Geometry: final body of the model. Coordinates: model frame, mm. A direction names the side the tool comes from. Coordinates: 2 decimals unless noted, no trailing zeros. Use CSV: the item, a comma, the result in double quotes. Start each with the question number.
Q1. Section query A-A, the plane y = -31. State how many separate pieces and enclosed holes the cut face has, and give its area (3 significant figures).
Q2. Mould query, pull axis X, two halves, no side actions, for faces 1 (the face through (3, 0, -3)), 2 (the face through (-67.5, -50, 2)), 3 (the face through (0, -10, 180)). Classes: +X half, -X half, draft (parallel to the pull), parting line (faces both ways), or undercut.
Q3. First-contact query: P1, Ø10, axis at y = -49.5, z = -59, coming from the -X side; P2, Ø18, axis at y = -44.5, z = -43, coming from the -X side; P3, Ø1.5, axis at x = 0.5, y = -54.5, coming from the -Z side. Flat tips, straight axial feed; report the tip coordinate or a pass-through.
Q4. Ray query, probe 1 along X at (y, z) = (-11.75, 0); probe 2 along X at (y, z) = (-9, -170). Return the intervals inside material, ascending.
Q5. Access query for faces 4 (the face through (-10, -10, -166)), 5 (the face through (-130.156, -49.58, 58.015)), 6 (the face through (87.5, -50, 2)), 7 (the face through (105.106, -9.86, -107.018)). Directions: +Z, -Z, +X, -X, +Y, -Y. A direction counts if a zero-diameter tool reaches every point of the face in a straight line with its end or side. Return the directions, or none.
from build123d import *

# Parameters (mm, degrees)
SKETCH3_R           = 5
BOSS_EXTRUDE4_DEPTH = 20
SKETCH4_W           = 5
SKETCH4_H           = 260
BOSS_EXTRUDE5_DEPTH = 60


with BuildPart() as part:
    # Sketch3 → Boss-Extrude4 (new body)
    with BuildSketch(Plane(origin=(0, 0, 0), x_dir=(1, 0, 0), z_dir=(0, 1, 0))):
        with BuildLine():
            Line((161.369142032, 10), (170, 10))
            ThreePointArc((170, 10), (180, 0), (170, -10))
            Line((170, -10), (161.369142032, -10))
            ThreePointArc((161.369142032, -10), (152.849946816, -13.180462695), (148.499210458, -21.165644172))
            ThreePointArc((148.499210458, -21.165644172), (106.066017178, -106.066017178), (21.165644172, -148.499210458))
            ThreePointArc((21.165644172, -148.499210458), (13.180462695, -152.849946816), (10, -161.369142032))
            Line((10, -161.369142032), (10, -170))
            ThreePointArc((10, -170), (0, -180), (-10, -170))
            Line((-10, -170), (-10, -161.369142032))
            ThreePointArc((-10, -161.369142032), (-13.180462695, -152.849946816), (-21.165644172, -148.499210458))
            ThreePointArc((-21.165644172, -148.499210458), (-106.066017178, -106.066017178), (-148.499210458, -21.165644172))
            ThreePointArc((-148.499210458, -21.165644172), (-152.849946816, -13.180462695), (-161.369142032, -10))
            Line((-161.369142032, -10), (-170, -10))
            ThreePointArc((-170, -10), (-180, 0), (-170, 10))
            Line((-170, 10), (-161.369142032, 10))
            ThreePointArc((-161.369142032, 10), (-152.849946816, 13.180462695), (-148.499210458, 21.165644172))
            ThreePointArc((-148.499210458, 21.165644172), (-106.066017178, 106.066017178), (-21.165644172, 148.499210458))
            ThreePointArc((-21.165644172, 148.499210458), (-13.180462695, 152.849946816), (-10, 161.369142032))
            Line((-10, 161.369142032), (-10, 170))
            ThreePointArc((-10, 170), (0, 180), (10, 170))
            Line((10, 170), (10, 161.369142032))
            ThreePointArc((10, 161.369142032), (13.180462695, 152.849946816), (21.165644172, 148.499210458))
            ThreePointArc((21.165644172, 148.499210458), (106.066017178, 106.066017178), (148.499210458, 21.165644172))
            ThreePointArc((148.499210458, 21.165644172), (152.849946816, 13.180462695), (161.369142032, 10))
        make_face()
        with Locations((0, 170)):
            Circle(SKETCH3_R, mode=Mode.SUBTRACT)
        with Locations((170, 0)):
            Circle(SKETCH3_R, mode=Mode.SUBTRACT)
        with Locations((0, -170)):
            Circle(SKETCH3_R, mode=Mode.SUBTRACT)
        with Locations((-170, 0)):
            Circle(SKETCH3_R, mode=Mode.SUBTRACT)
    extrude(amount=-BOSS_EXTRUDE4_DEPTH)

    # Sketch4 → Boss-Extrude5 (add)
    with BuildSketch(Plane(origin=(0, -20, 0), x_dir=(1, 0, 0), z_dir=(0, 1, 0))):
        Rectangle(SKETCH4_W, SKETCH4_H)
        with Locations((10, 0)):
            Rectangle(SKETCH4_W, SKETCH4_H)
        with Locations((20, 0)):
            Rectangle(SKETCH4_W, SKETCH4_H)
        with Locations((30, 0)):
            Rectangle(SKETCH4_W, SKETCH4_H)
        with Locations((40, 0)):
            Rectangle(SKETCH4_W, SKETCH4_H)
        with Locations((50, 0)):
            Rectangle(SKETCH4_W, SKETCH4_H)
        with Locations((60, 0)):
            Rectangle(SKETCH4_W, SKETCH4_H)
        with Locations((70, 0)):
            Rectangle(SKETCH4_W, SKETCH4_H)
        with BuildLine():
            Line((82.5, 116.189500386), (82.5, -116.189500386))
            ThreePointArc((82.5, -116.189500386), (80.017987314, -117.912559578), (77.5, -119.582607431))
            Line((77.5, -119.582607431), (77.5, 119.582607431))
            ThreePointArc((77.5, 119.582607431), (80.017987314, 117.912559578), (82.5, 116.189500386))
        make_face()
        with BuildLine():
            Line((92.5, 108.397416943), (92.5, -108.397416943))
            ThreePointArc((92.5, -108.397416943), (90.023058171, -110.463111478), (87.5, -112.472218792))
            Line((87.5, -112.472218792), (87.5, 112.472218792))
            ThreePointArc((87.5, 112.472218792), (90.023058171, 110.463111478), (92.5, 108.397416943))
        make_face()
        with BuildLine():
            Line((102.5, 98.994949366), (102.5, -98.994949366))
            ThreePointArc((102.5, -98.994949366), (100.030353094, -101.489794856), (97.5, -103.923048454))
            Line((97.5, -103.923048454), (97.5, 103.923048454))
            ThreePointArc((97.5, 103.923048454), (100.030353094, 101.489794856), (102.5, 98.994949366))
        make_face()
        with BuildLine():
            Line((112.5, 87.464278423), (112.5, -87.464278423))
            ThreePointArc((112.5, -87.464278423), (110.041959984, -90.537379258), (107.5, -93.541434669))
            Line((107.5, -93.541434669), (107.5, 93.541434669))
            ThreePointArc((107.5, 93.541434669), (110.041959984, 90.537379258), (112.5, 87.464278423))
        make_face()
        with Locations((-10, 0)):
            Rectangle(SKETCH4_W, SKETCH4_H)
        with Locations((-20, 0)):
            Rectangle(SKETCH4_W, SKETCH4_H)
        with Locations((-30, 0)):
            Rectangle(SKETCH4_W, SKETCH4_H)
        with Locations((-40, 0)):
            Rectangle(SKETCH4_W, SKETCH4_H)
        with Locations((-50, 0)):
            Rectangle(SKETCH4_W, SKETCH4_H)
        with Locations((-60, 0)):
            Rectangle(SKETCH4_W, SKETCH4_H)
        with Locations((-70, 0)):
            Rectangle(SKETCH4_W, SKETCH4_H)
        with BuildLine():
            Line((-82.5, 116.189500386), (-82.5, -116.189500386))
            ThreePointArc((-82.5, -116.189500386), (-80.017987314, -117.912559578), (-77.5, -119.582607431))
            Line((-77.5, -119.582607431), (-77.5, 119.582607431))
            ThreePointArc((-77.5, 119.582607431), (-80.017987314, 117.912559578), (-82.5, 116.189500386))
        make_face()
        with BuildLine():
            Line((-92.5, 108.397416943), (-92.5, -108.397416943))
            ThreePointArc((-92.5, -108.397416943), (-90.023058171, -110.463111478), (-87.5, -112.472218792))
            Line((-87.5, -112.472218792), (-87.5, 112.472218792))
            ThreePointArc((-87.5, 112.472218792), (-90.023058171, 110.463111478), (-92.5, 108.397416943))
        make_face()
        with BuildLine():
            Line((-102.5, 98.994949366), (-102.5, -98.994949366))
            ThreePointArc((-102.5, -98.994949366), (-100.030353094, -101.489794856), (-97.5, -103.923048454))
            Line((-97.5, -103.923048454), (-97.5, 103.923048454))
            ThreePointArc((-97.5, 103.923048454), (-100.030353094, 101.489794856), (-102.5, 98.994949366))
        make_face()
        with BuildLine():
            Line((-112.5, 87.464278423), (-112.5, -87.464278423))
            ThreePointArc((-112.5, -87.464278423), (-110.041959984, -90.537379258), (-107.5, -93.541434669))
            Line((-107.5, -93.541434669), (-107.5, 93.541434669))
            ThreePointArc((-107.5, 93.541434669), (-110.041959984, 90.537379258), (-112.5, 87.464278423))
        make_face()
        with BuildLine():
            Line((-122.5, 72.801098893), (-122.5, -72.801098893))
            ThreePointArc((-122.5, -72.801098893), (-120.063707597, -76.752564245), (-117.5, -80.622577483))
            Line((-117.5, -80.622577483), (-117.5, 80.622577483))
            ThreePointArc((-117.5, 80.622577483), (-120.063707597, 76.752564245), (-122.5, 72.801098893))
        make_face()
        with BuildLine():
            Line((-132.5, 52.440442409), (-132.5, -52.440442409))
            ThreePointArc((-132.5, -52.440442409), (-130.120541577, -58.09384356), (-127.5, -63.639610307))
            Line((-127.5, -63.639610307), (-127.5, 63.639610307))
            ThreePointArc((-127.5, 63.639610307), (-130.120541577, 58.09384356), (-132.5, 52.440442409))
        make_face()
        with BuildLine():
            Line((-137.5, 37.416573868), (-137.5, -37.416573868))
            ThreePointArc((-137.5, -37.416573868), (-142.5, 0), (-137.5, 37.416573868))
        make_face()
        with BuildLine():
            Line((122.5, 72.801098893), (122.5, -72.801098893))
            ThreePointArc((122.5, -72.801098893), (120.063707597, -76.752564245), (117.5, -80.622577483))
            Line((117.5, -80.622577483), (117.5, 80.622577483))
            ThreePointArc((117.5, 80.622577483), (120.063707597, 76.752564245), (122.5, 72.801098893))
        make_face()
        with BuildLine():
            Line((132.5, 52.440442409), (132.5, -52.440442409))
            ThreePointArc((132.5, -52.440442409), (130.120541577, -58.09384356), (127.5, -63.639610307))
            Line((127.5, -63.639610307), (127.5, 63.639610307))
            ThreePointArc((127.5, 63.639610307), (130.120541577, 58.09384356), (132.5, 52.440442409))
        make_face()
        with BuildLine():
            Line((137.5, 37.416573868), (137.5, -37.416573868))
            ThreePointArc((137.5, -37.416573868), (142.5, 0), (137.5, 37.416573868))
        make_face()
    extrude(amount=-BOSS_EXTRUDE5_DEPTH)


solid = part.part
Responses:
1,separate pieces,"29"
1,enclosed holes,"0"
1,area,"31,100 mm²"
2,face 1,"draft"
2,face 2,"undercut"
2,face 3,"parting line"
3,P1,"stops at x = -131.87"
3,P2,"stops at x = -138.38"
3,P3,"stops at z = -130"
4,probe 1,"x = -180 to -175, -165 to 165, 175 to 180"
4,probe 2,"x = -10 to -5, 5 to 10"
5,face 4,"-Z, -X, +Y, -Y"
5,face 5,"+Z, -X, -Y"
5,face 6,"+Z, -Z, -Y"
5,face 7,"-Z, +X, +Y, -Y"
